Could you check a few things on this model? Use its own coordinates, in mm. A direction names the side the tool comes from. Give positions to 0.01 mm unless a question says otherwise; leave off trailing zeros. Write each loop counter-clockwise with the first axis right and the second up, starting at its lowest first coordinate (ties: lowest second). Pieces come first, ordered by that corner, then holes. Notation, with made-up numbers: M 69,-6.75 L 120,-6.75 A22 ccw 120,31.25 Z; hole C 48,42.25 d9. An arc over 180 degrees is marked long. One line per item, written item: value.
Autodesk Inventor part; units mm, degrees
ref_plane "YZ Plane" through (0, 0, 0) normal (1, 0, 0) x (0, 1, 0)
ref_plane "XZ Plane" through (0, 0, 0) normal (0, 1, 0) x (-1, 0, 0)
ref_plane "XY Plane" through (0, 0, 0) normal (0, 0, 1) x (1, 0, 0)
sketch "Sketch1" plane through (0, 0, 0) normal (0, 1, 0) x (-1, 0, 0)
  line L0 (0, 0) -> (-99, 0)
  line L1 (-99, 0) -> (-99, -48)
  line L2 (-99, -48) -> (0, -48)
  line L3 (0, -48) -> (0, 0)
  dimension "d0" = 99
  dimension "d1" = 48
extrude "Extrusion1" add sketch "Sketch1" along normal blind 4
sketch "Sketch2" plane through (0, 4, 0) normal (0, 1, 0) x (1, 0, 0)
  line L0 (99, 48) -> (0, 48) construction
  line L1 (99, 0) -> (99, 48) construction
  line L2 (0, 0) -> (99, 0) construction
  line L3 (0, 48) -> (0, 0) construction
  line L4 (4, 44) -> (95, 44) construction
  line L5 (95, 44) -> (95, 4) construction
  line L6 (95, 4) -> (4, 4) construction
  line L7 (4, 4) -> (4, 44) construction
  line L8 (4, 36) -> (0, 36)
  line L9 (0, 36) -> (0, 48)
  line L10 (0, 48) -> (4, 48)
  line L11 (4, 48) -> (4, 36)
  line L12 (0, 24) -> (99, 24) construction
  line L13 (49.5, 0) -> (49.5, 48) construction
  line L14 (0, 28) -> (4, 28)
  line L15 (0, 28) -> (0, 24)
  line L16 (4, 28) -> (4, 24)
  line L17 (13.5, 48) -> (13.5, 44)
  line L18 (13.5, 44) -> (21.5, 44)
  line L19 (21.5, 44) -> (21.5, 48)
  line L20 (21.5, 48) -> (13.5, 48)
  line L21 (29.5, 48) -> (29.5, 44)
  line L22 (29.5, 44) -> (37.5, 44)
  line L23 (37.5, 48) -> (37.5, 44)
  line L24 (37.5, 48) -> (29.5, 48)
  line L25 (45.5, 44) -> (45.5, 48)
  line L26 (45.5, 44) -> (49.5, 44)
  line L27 (49.5, 48) -> (45.5, 48)
  line L28 (4, 12) -> (0, 12)
  line L29 (0, 12) -> (0, 0)
  line L30 (0, 0) -> (4, 0)
  line L31 (4, 0) -> (4, 12)
  line L32 (0, 20) -> (4, 20)
  line L33 (0, 20) -> (0, 24)
  line L34 (4, 20) -> (4, 24)
  line L35 (13.5, 0) -> (13.5, 4)
  line L36 (13.5, 4) -> (21.5, 4)
  line L37 (21.5, 4) -> (21.5, 0)
  line L38 (21.5, 0) -> (13.5, 0)
  line L39 (29.5, 0) -> (29.5, 4)
  line L40 (29.5, 4) -> (37.5, 4)
  line L41 (37.5, 0) -> (37.5, 4)
  line L42 (37.5, 0) -> (29.5, 0)
  line L43 (45.5, 4) -> (45.5, 0)
  line L44 (45.5, 4) -> (49.5, 4)
  line L45 (49.5, 0) -> (45.5, 0)
  line L46 (99, 48) -> (99, 0) construction
  line L47 (95, 4) -> (95, 44) construction
  line L48 (95, 36) -> (99, 36)
  line L49 (99, 36) -> (99, 48)
  line L50 (99, 48) -> (95, 48)
  line L51 (95, 48) -> (95, 36)
  line L52 (99, 28) -> (95, 28)
  line L53 (99, 28) -> (99, 24)
  line L54 (95, 28) -> (95, 24)
  line L55 (85.5, 48) -> (85.5, 44)
  line L56 (85.5, 44) -> (77.5, 44)
  line L57 (77.5, 44) -> (77.5, 48)
  line L58 (77.5, 48) -> (85.5, 48)
  line L59 (69.5, 48) -> (69.5, 44)
  line L60 (69.5, 44) -> (61.5, 44)
  line L61 (61.5, 48) -> (61.5, 44)
  line L62 (61.5, 48) -> (69.5, 48)
  line L63 (53.5, 44) -> (53.5, 48)
  line L64 (53.5, 44) -> (49.5, 44)
  line L65 (49.5, 48) -> (53.5, 48)
  line L66 (99, 0) -> (95, 0)
  line L67 (69.5, 0) -> (69.5, 4)
  line L68 (69.5, 4) -> (61.5, 4)
  line L69 (61.5, 0) -> (69.5, 0)
  line L70 (61.5, 0) -> (61.5, 4)
  line L71 (53.5, 4) -> (53.5, 0)
  line L72 (53.5, 4) -> (49.5, 4)
  line L73 (49.5, 0) -> (53.5, 0)
  line L74 (95, 0) -> (95, 12)
  line L75 (95, 12) -> (99, 12)
  line L76 (99, 12) -> (99, 0)
  line L77 (85.5, 0) -> (85.5, 4)
  line L78 (99, 20) -> (95, 20)
  line L79 (77.5, 0) -> (85.5, 0)
  line L80 (77.5, 4) -> (77.5, 0)
  line L81 (85.5, 4) -> (77.5, 4)
  line L82 (95, 20) -> (95, 24)
  line L83 (99, 20) -> (99, 24)
  dimension "d8" = 4
  dimension "d11" = 8
  dimension "d12" = 4
  dimension "d14" = 8
  dimension "d15" = 8
  dimension "d16" = 8
  dimension "d17" = 4
  dimension "d18" = 8
extrude "Extrusion2" cut sketch "Sketch2" against normal up to surface (4 mm away)
sketch "Sketch3" plane through (0, 4, 0) normal (0, 1, 0) x (1, 0, 0)
  line L0 (4, 12) -> (4, 0)
  line L1 (4, 12) -> (95, 12)
  line L2 (95, 12) -> (95, 20)
  line L3 (95, 20) -> (4, 20)
  line L4 (4, 20) -> (4, 12)
  line L5 (13.5, 4) -> (21.5, 4)
  point P0 (0, 0)
  dimension "d21" = 8
  dimension "d22" = 8
extrude "Extrusion3" add sketch "Sketch3" along normal blind 3
properties part number "front" material "PBT Plastic Black"
1) If we section it at C-C, the plane y = 5.25: Write out the boundary of the cut face in (x, z), then the cut area to 3 significant figures.
Outcome:
outline: M 4,-20 L 95,-20 L 95,-12 L 4,-12 Z
area: 728 mm^2
2) I'm going to push flat-ended pins straight in: pin 1 (2 mm diameter, centred on y = 3, z = -46.5, fed in from +X); pin 2 (1.2 mm diameter, centred on y = 1.5, z = -47, fed in from -X); pin 3 (4 mm diameter, centred on x = 82.5, y = 5, fed in from -Z); pin 4 (6 mm diameter, centred on x = 73.5, z = -10.5, fed in from +Y). Where does each tip first touch, or does it pass through?
Outcome:
pin 1: stops at x = 95
pin 2: stops at x = 4
pin 3: stops at z = -44
pin 4: stops at y = 7
3) If we section it at A-A, the plane z = -14.5: Write out the boundary of the cut face in (x, y), then the cut area to 3 significant figures.
Outcome:
outline: M 0,0 L 99,0 L 99,4 L 95,4 L 95,7 L 4,7 L 4,4 L 0,4 Z
area: 669 mm^2
4) If we section it at D-D, the plane z = -24.5: Write out the boundary of the cut face in (x, y), then the cut area to 3 significant figures.
Outcome:
outline: M 4,0 L 95,0 L 95,4 L 4,4 Z
area: 364 mm^2
5) We'd pull the mould along X, two halves only. Please class faces 5 (the face through (50, 5, -20)), 6 (the face through (4, 2, -6)), 7 (the face through (50, 2, -44)): pulls with the +X half, pulls with the -X half, needs draft (parallel to the pull), parting line crosses it, or undercut.
Outcome:
face 5: needs draft
face 6: pulls with the -X half
face 7: undercut
6) If we section it at B-B, the plane x = 32: Write out the boundary of the cut face in (y, z).
Outcome:
outline: M 0,-44 L 4,-44 L 4,-20 L 7,-20 L 7,-12 L 4,-12 L 4,-4 L 0,-4 Z
7) On a 3-axis mill with a long thin cutter (end or side, diameter ignored), from which of +Z, -Z, +X, -X, +Y, -Y can I reach the whole of each face in a straight line? I mean faces 1 (the face through (49, 5, -12)), 2 (the face through (82, 2, -44)), 3 (the face through (82, 2, -4)), 4 (the face through (4, 2, -42)). Say none if no direction works.
Outcome:
face 1: +Z, +X, -X, +Y
face 2: -Z, +Y, -Y
face 3: +Z, +Y, -Y
face 4: -Z, -X, +Y, -Y
8) Please list where these lines run through material, in increasing order: L1, parallel to Y at x = 62.5, z = -11; L2, parallel to Z at x = 50, y = 6.25; L3, parallel to Z at x = 63, y = 3.5. Write a range as from..to.
Outcome:
L1: y = 0..4
L2: z = -20..-12
L3: z = -44..-4
